Here's how the part is built. I have some questions about the finished solid (model axes, mm). A direction names the side the tool comes from. Round coordinates to 2 decimals unless told otherwise and drop trailing zeros. Write each loop counter-clockwise with the first axis right and the second up, starting at its lowest first coordinate (ties: lowest second). Pieces come first, ordered by that corner, then holes. Notation, with made-up numbers: (72.25, 14) - (91.25, 14) arc R18 ccw to (91.25, 26) - close; hole circle Ø4 at (75.5, -8). An arc over 180 degrees is marked (long way). One line per item, written item: value. Start each with the question number.
Item 1: For P1, Ø1, axis at y = 55.5, z = -11, coming from the +X side; P2, Ø1, axis at x = 37, z = -27, coming from the -Y side; P3, Ø6, axis at y = 12.5, z = -8.5, coming from the +X side, each with a flat end and sliding along its axis, tell me the tip position at first contact or that it passes through.
Item 2: For faces 5 (the face through (122.91, 42, -1.2)), 6 (the face through (8.07, 40.45, -54.7)), 7 (the face through (95.25, 16.99, -56.52)), which set-ups out of +Z, -Z, +X, -X, +Y, -Y let a thin tool reach every point of the face, with its end or its side?
Item 3: Imagine slicing it at C-C, the plane x = 64.5. Please give me the cut outline in (y, z).
Item 4: Imagine slicing it at D-D, the plane x = 21. Please give me the cut outline in (y, z).
Item 5: Thinking about a two-plate mould opening in Z: for faces 1 (the face through (6.15, 41.99, -1.14)), 2 (the face through (120.92, 40.45, -54.71)), 3 (the face through (6.09, 42, -56.8)), 4 (the face through (65, 85, -29)), which applies, released by +Z, released by -Z, zero draft, split by the parting line, or undercut?
Item 6: Imagine slicing it at B-B, the plane z = -34.5. Please give me the cut outline in (x, y), then the cut area to 3 significant figures.
Item 7: Imagine slicing it at A-A, the plane x = 102.5. Please give me the cut outline in (y, z).
Item 8: If I drill on line 1 (Z direction, x = 38, y = 63); line 2 (X direction, y = 20, z = -56.2); line 3 (Y direction, x = 64.5, z = -56.5), over which ranges is the centre line in solid material (lowest first)?
Autodesk Inventor part; units mm, degrees
ref_plane "YZ Plane" through (0, 0, 0) normal (1, 0, 0) x (0, 1, 0)
ref_plane "XZ Plane" through (0, 0, 0) normal (0, 1, 0) x (-1, 0, 0)
ref_plane "XY Plane" through (0, 0, 0) normal (0, 0, 1) x (1, 0, 0)
sketch "Sketch1" plane through (0, 0, 0) normal (0, 0, 1) x (1, 0, 0)
  line L0 (0, 0) -> (129, 0)
  line L1 (129, 0) -> (129, 85)
  line L2 (129, 85) -> (0, 85)
  line L3 (0, 85) -> (0, 0)
  line L4 (0, 85) -> (10, 85)
  line L5 (10, 85) -> (0, 0)
  line L6 (129, 85) -> (119, 85)
  line L7 (119, 85) -> (129, 0)
  dimension "d0" = 129
  dimension "d1" = 85
  dimension "d2" = 10
  dimension "d3" = 10
extrude "Extrusion1" add sketch "Sketch1" against normal blind 58 contours L5 L2 L7 L0
fillet "Fillet1" radius 4 4 edges at (5, 42.5, 0) (124, 42.5, 0) (124, 42.5, -58) (5, 42.5, -58)
shell "Shell1" thickness 3 removed faces 1 at (44.3425, 0, -19.3333)
sketch "Sketch3" plane through (0, 0, -58) normal (0, 0, -1) x (-1, 0, 0)
  line L0 (-14.0276, 85) -> (-114.9724, 85)
  line L1 (-124.9724, 0) -> (-4.0276, 0)
  line L2 (-64.5, 0) -> (-64.5, 85)
  line L3 (-64.5, 85) -> (-64.5, 55)
  circle A0 centre (-64.5, 55) radius 22.5
  line L4 (-64.5, 0) -> (-102.5, 0)
  line L5 (-102.5, 0) -> (-102.5, 20)
  line L6 (-102.5, 20) -> (-64.5, 20)
  line L7 (-64.5, 20) -> (-64.5, 0)
  line L8 (-64.5, 0) -> (-26.5, 0)
  line L9 (-26.5, 0) -> (-26.5, 20)
  line L10 (-26.5, 20) -> (-64.5, 20)
  line L11 (-64.5, 20) -> (-64.5, 0)
  circle A1 centre (-26.5, 20) radius 7.85
  circle A2 centre (-102.5, 20) radius 7.85
  point P0 (0, 0)
  dimension "d18" = 30
  dimension "d19" = 45
  dimension "d20" = 38
  dimension "d21" = 20
  dimension "d22" = 38
  dimension "d23" = 15.7
  dimension "d24" = 15.7
extrude "Extrusion3" cut sketch "Sketch3" against normal blind 10 contours A0 L2 | L2 A0 | A2 L6 L5 | L5 L6 A2 | A1 L10 L9 | L9 L10 A1
chamfer "Chamfer1" distance 3 distance2 1 1 edges at (87, 55, -58) measured on face at (52.7612, 4.22, -58)
properties part number "Box MKIV Version 2"
Values follow:
1. P1: stops at x = 122.53
1. P2: stops at y = 82
1. P3: stops at x = 127.88
2. face 5: +Z, +X, +Y
2. face 6: -Y
2. face 7: -Z
3. outline: (0, -58) - (29.5, -58) - (32.5, -57) - (32.5, -55) - (0, -55) - close; (0, -3) - (82, -3) - (82, -55) - (77.5, -55) - (77.5, -57) - (80.5, -58) - (85, -58) - (85, 0) - (0, 0) - close
4. outline: (0, -58) - (14.4, -58) - (14.4, -55) - (0, -55) - close; (0, -3) - (82, -3) - (82, -55) - (25.6, -55) - (25.6, -58) - (85, -58) - (85, 0) - (0, 0) - close
5. face 1: released by +Z
5. face 2: undercut
5. face 3: released by -Z
5. face 4: zero draft
6. outline: (0, 0) - (3.02, 0) - (12.67, 82) - (116.33, 82) - (125.98, 0) - (129, 0) - (119, 85) - (10, 85) - close
6. area: 823 mm^2
7. outline: (0, -58) - (12.15, -58) - (12.15, -55) - (0, -55) - close; (0, -3) - (82, -3) - (82, -55) - (27.85, -55) - (27.85, -58) - (85, -58) - (85, 0) - (0, 0) - close
8. line 1: z = -58 to -55, -3 to 0
8. line 2: x = 3.02 to 18.65, 34.35 to 94.65, 110.35 to 125.98
8. line 3: y = 0 to 32.5, 77.5 to 85
